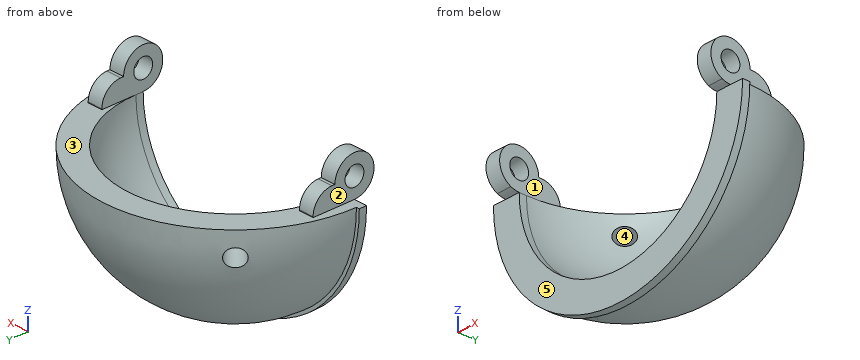
from build123d import *

# Parameters (mm, degrees)
BOSS_EXTRUDE1_DEPTH              = 1.27
REVOLVE3_ANGLE                   = 90
SKETCH6_W                        = 4.862612613
SKETCH6_H                        = 1.27
BOSS_EXTRUDE3_DEPTH              = 7.935530078
BOSS_EXTRUDE4_DEPTH              = 3.81
BOSS_EXTRUDE4_DEPTH_BACK         = 6.35
SKETCH10_W                       = 4.862612613
SKETCH10_H                       = 7.935530078
FILLET7_R                        = 5.08
FILLET10_R                       = 5.08
SKETCH13_R                       = 1.651
CUT_EXTRUDE2_DEPTH               = 55.372
SKETCH14_W                       = 2.286
SKETCH14_H                       = 11.368095807
CUT_EXTRUDE3_DEPTH               = 55.372
FILLET15_RADIUS                  = 3.967765039
FILLET15_LENGTH                  = 2.576612613
FILLET16_RADIUS                  = 3.967765039
FILLET16_LENGTH                  = 2.576612613
CUT_EXTRUDE4_DEPTH               = 55.372
CUT_EXTRUDE7_DEPTH               = 55.88
SKETCH19_W                       = 2.576612613
SKETCH19_H                       = 3.428576371
BOSS_EXTRUDE5_DEPTH              = 3.81
FILLET17_R                       = 3.302
FILLET18_R                       = 3.302
F_96_0_0063_DIAMETER_HOLE2_D     = 3.302
F_96_0_0063_DIAMETER_HOLE2_DEPTH = 25.4
F_96_0_0063_DIAMETER_HOLE2_TIP   = 0.992020882


with BuildPart() as part:
    # Sketch1 → Boss-Extrude1 (new body)
    with BuildSketch(Plane(origin=(0, 0, 0), x_dir=(1, 0, 0), z_dir=(0, 1, 0))):
        with BuildLine():
            Line((-18.44626818, 0), (-13.583655567, 0))
            ThreePointArc((-13.583655567, 0), (5.056359448, 18.640015015), (23.696374463, 0))
            Line((23.696374463, 0), (28.558987076, 0))
            ThreePointArc((28.558987076, 0), (5.056359448, 23.502627628), (-18.44626818, 0))
        make_face()
    extrude(amount=BOSS_EXTRUDE1_DEPTH)

    # Sketch4 → Revolve3 (revolve)
    with BuildSketch(Plane(origin=(0, 1.27, 0), x_dir=(1, 0, 0), z_dir=(0, 1, 0))):
        with BuildLine():
            Line((23.696374463, 0), (28.014374463, 0))
            ThreePointArc((28.014374463, 0), (5.056359448, 22.958015015), (-17.901655567, 0))
            Line((-17.901655567, 0), (-13.583655567, 0))
            ThreePointArc((-13.583655567, 0), (5.056359448, 18.640015015), (23.696374463, 0))
        make_face()
    revolve(axis=Axis((-17.901655567, 1.27, 0), (1, 0, 0)), revolution_arc=REVOLVE3_ANGLE)

    # Sketch6 → Boss-Extrude3 (add)
    with BuildSketch(Plane.XY):
        with Locations((-16.014961873, 0.635)):
            Rectangle(SKETCH6_W, SKETCH6_H)
        with Locations((26.12768077, 0.635)):
            Rectangle(SKETCH6_W, SKETCH6_H)
    extrude(amount=BOSS_EXTRUDE3_DEPTH)

    # Sketch10 → Boss-Extrude4 (add, two sides: drawn at the far end of the back side and taken through both)
    with BuildSketch(Plane(origin=(0, 1.27, 0), x_dir=(1, 0, 0), z_dir=(0, 1, 0)).offset(-BOSS_EXTRUDE4_DEPTH_BACK)):
        with Locations((-16.014961873, -3.967765039)):
            Rectangle(SKETCH10_W, SKETCH10_H)
        with Locations((26.12768077, -3.967765039)):
            Rectangle(SKETCH10_W, SKETCH10_H)
    extrude(amount=BOSS_EXTRUDE4_DEPTH + BOSS_EXTRUDE4_DEPTH_BACK)

    # Fillet7
    fillet7_edges = [part.edges().sort_by_distance(p)[0] for p in [
        (-16.014961873, 5.08, 7.935530078),
    ]]
    fillet(fillet7_edges, radius=FILLET7_R)

    # Fillet10
    fillet10_edges = [part.edges().sort_by_distance(p)[0] for p in [
        (26.127680769, 5.08, 7.935530078),
    ]]
    fillet(fillet10_edges, radius=FILLET10_R)

    # Sketch13 → Cut-Extrude2 (cut)
    with BuildSketch(Plane.ZY.offset(18.44626818)):
        with Locations((3.428576371, 0)):
            Circle(SKETCH13_R)
    extrude(amount=-CUT_EXTRUDE2_DEPTH, mode=Mode.SUBTRACT)

    # Sketch14 → Cut-Extrude3 (cut)
    with BuildSketch(Plane(origin=(0, 5.08, 0), x_dir=(1, 0, 0), z_dir=(0, 1, 0))):
        with Locations((27.415987076, -5.684047904)):
            Rectangle(SKETCH14_W, SKETCH14_H)
        with Locations((-17.30326818, -5.684047904)):
            Rectangle(SKETCH14_W, SKETCH14_H)
    extrude(amount=-CUT_EXTRUDE3_DEPTH, mode=Mode.SUBTRACT)

    # Fillet15: full round fillet: the end face becomes a half cylinder, R = half its width
    fillet15_face = Plane((24.984680769, -5.08, 3.967765039), x_dir=(1, 0, 0), z_dir=(0, -1, 0))  # on the end face: x along it, z out of the body
    fillet15_slab = fillet15_face.offset(-FILLET15_RADIUS / 2) * Box(FILLET15_LENGTH, 2 * FILLET15_RADIUS, FILLET15_RADIUS, mode=Mode.PRIVATE)  # the body's end, R deep
    fillet15_round = Plane((24.984680769, -1.112234961, 3.967765039), x_dir=(0, -1, 0), z_dir=(1, 0, 0)) * Cylinder(FILLET15_RADIUS, FILLET15_LENGTH, mode=Mode.PRIVATE)  # its axis R under the face
    add(fillet15_slab - fillet15_round, mode=Mode.SUBTRACT)

    # Fillet16: full round fillet: the end face becomes a half cylinder, R = half its width
    fillet16_face = Plane((-14.871961873, -5.08, 3.967765039), x_dir=(-1, 0, 0), z_dir=(0, -1, 0))  # on the end face: x along it, z out of the body
    fillet16_slab = fillet16_face.offset(-FILLET16_RADIUS / 2) * Box(FILLET16_LENGTH, 2 * FILLET16_RADIUS, FILLET16_RADIUS, mode=Mode.PRIVATE)  # the body's end, R deep
    fillet16_round = Plane((-14.871961873, -1.112234961, 3.967765039), x_dir=(0, -1, 0), z_dir=(-1, 0, 0)) * Cylinder(FILLET16_RADIUS, FILLET16_LENGTH, mode=Mode.PRIVATE)  # its axis R under the face
    add(fillet16_slab - fillet16_round, mode=Mode.SUBTRACT)

    # Sketch16 → Cut-Extrude4 (cut)
    with BuildSketch(Plane(origin=(26.272987076, 0, 0), x_dir=(0, 0, -1), z_dir=(1, 0, 0))):
        with BuildLine():
            ThreePointArc((0, 0), (-3.716578938, -3.862364093), (-7.935530078, -0.55611748))
            ThreePointArc((-7.935530078, -0.55611748), (-3.630565744, -5.089731167), (0, 0))
        make_face()
    extrude(amount=-CUT_EXTRUDE4_DEPTH, mode=Mode.SUBTRACT)

    # Sketch18 → Cut-Extrude7 (cut)
    with BuildSketch(Plane(origin=(26.272987076, 0, 0), x_dir=(0, 0, -1), z_dir=(1, 0, 0))):
        with BuildLine():
            Line((-3.428576371, 3.428576371), (0, 3.428576371))
            Line((0, 3.428576371), (0, 5.467356317))
            Line((0, 5.467356317), (-9.031573881, 5.467356317))
            Line((-9.031573881, 5.467356317), (-9.031573881, -4.486785293))
            Line((-9.031573881, -4.486785293), (0, -4.486785293))
            Line((0, -4.486785293), (0, 0))
            ThreePointArc((0, 0), (-5.852945973, -2.424369602), (-3.428576371, 3.428576371))
        make_face()
    extrude(amount=-CUT_EXTRUDE7_DEPTH, mode=Mode.SUBTRACT)

    # Sketch19 → Boss-Extrude5 (add)
    with BuildSketch(Plane(origin=(0, 3.428576371, 0), x_dir=(1, 0, 0), z_dir=(0, 1, 0))):
        with Locations((24.98468077, -1.714288186)):
            Rectangle(SKETCH19_W, SKETCH19_H)
        with Locations((-14.871961874, -1.714288186)):
            Rectangle(SKETCH19_W, SKETCH19_H)
    extrude(amount=BOSS_EXTRUDE5_DEPTH)

    # Fillet17
    fillet17_edges = [part.edges().sort_by_distance(p)[0] for p in [
        (24.984680769, 7.238576371, 3.428576371),
    ]]
    fillet(fillet17_edges, radius=FILLET17_R)

    # Fillet18
    fillet18_edges = [part.edges().sort_by_distance(p)[0] for p in [
        (-14.871961873, 7.238576371, 3.428576371),
    ]]
    fillet(fillet18_edges, radius=FILLET18_R)

    # #96 (0.0063) Diameter Hole2
    with Locations(Plane(origin=(-11.529605698, 16.548146571, -4.307487778), x_dir=(-0.677514134429, -0.735509753605, 0), z_dir=(-0.722447700093, 0.665482035826, -0.187624573613))):
        with Locations((0, 0)):
            Hole(F_96_0_0063_DIAMETER_HOLE2_D / 2, depth=F_96_0_0063_DIAMETER_HOLE2_DEPTH)
            with Locations((0, 0, -(F_96_0_0063_DIAMETER_HOLE2_DEPTH + F_96_0_0063_DIAMETER_HOLE2_TIP / 2))):  # 118° drill point
                Cone(0, F_96_0_0063_DIAMETER_HOLE2_D / 2, F_96_0_0063_DIAMETER_HOLE2_TIP, mode=Mode.SUBTRACT)


solid = part.part
Can you work these out from the model? Positions are in its coordinate system, mm. Face numbers are marked on the shaded views. A direction names the side the tool comes from. Give positions to 0.01 mm unless a question says otherwise; leave off trailing zeros. Order: outer loops, then holes, each group sorted by start corner. A loop starts at its lowest first (then second) coordinate and runs counter-clockwise, first axis right, second up. Notation, with made-up numbers: M 55.25,47.5 L 66.25,47.5 A19 ccw 66.25,81.5 Z; hole C 65.5,5 d3. An arc over 180 degrees is marked long. Use one line per item in the form item = value.
Item 1: If I drill on line 1 along Y through (x, z) = (25, 3); line 2 along X through (y, z) = (3, -3); line 3 along Z through (x, y) = (-3, 7), over which ranges is the centre line in solid material (lowest first)? Write a range as [from, to].
Values follow:
line_1 = [-3.4, -1.59], [1.59, 5.56]
line_2 = [-17.64, -13.26], [23.37, 27.75]
line_3 = [-20.72, -15.8]
Item 2: If we section it at B-B, the plane x = 1: Write out the boundary of the cut face in (y, z).
Values follow:
outline = M 0,-23.15 L 1.27,-23.15 L 1.27,-22.6 A22.6 ccw 23.87,0 L 19.46,0 A18.19 cw 1.27,-18.19 L 0,-18.19 Z
Item 3: If we section it at A-A, the plane z = 1: Write out the boundary of the cut face in (x, y), and give its area (3 significant figures).
Values follow:
outline = M -16.16,-2.42 L -13.58,-2.42 L -13.58,7.12 L -16.16,7.12 Z; M 23.7,-2.42 L 26.27,-2.42 L 26.27,7.12 L 23.7,7.12 Z
area = 49.2 mm^2
Item 4: If we section it at D-D, the plane y = 8.5: Write out the boundary of the cut face in (x, z).
Values follow:
outline = M -16.73,0 A21.79 ccw 26.85,0 L 22.24,0 A17.18 cw -12.12,0 Z
Item 5: Will these pins go through, and if not, where does the flat tip stop? pin 1 Ø4 at (x, y) = (3.5, 5.5) entering from +Z; pin 2 Ø4 at (y, z) = (2.5, -6.5) entering from -X; pin 3 Ø7.5 at (y, z) = (3.5, 5) entering from -X.
Values follow:
pin_1 = -17.47
pin_2 = -17.92
pin_3 = -16.16
Item 6: For the marked faces 1 and 2, which set-ups out of +Z, -Z, +X, -X, +Y, -Y let a thin tool reach every point of the face, with its end or its side?
Values follow:
face_1 = +Z, +Y, -Y
face_2 = +Z, -X, +Y, -Y
Item 7: Thinking about a two-plate mould opening in Y: for the marked faces 3, 4 and 5, which applies, pulls with the +Y half, pulls with the -Y half, needs draft (parallel to the pull), parting line crosses it, or undercut?
Values follow:
face_3 = needs draft
face_4 = undercut
face_5 = pulls with the -Y half
